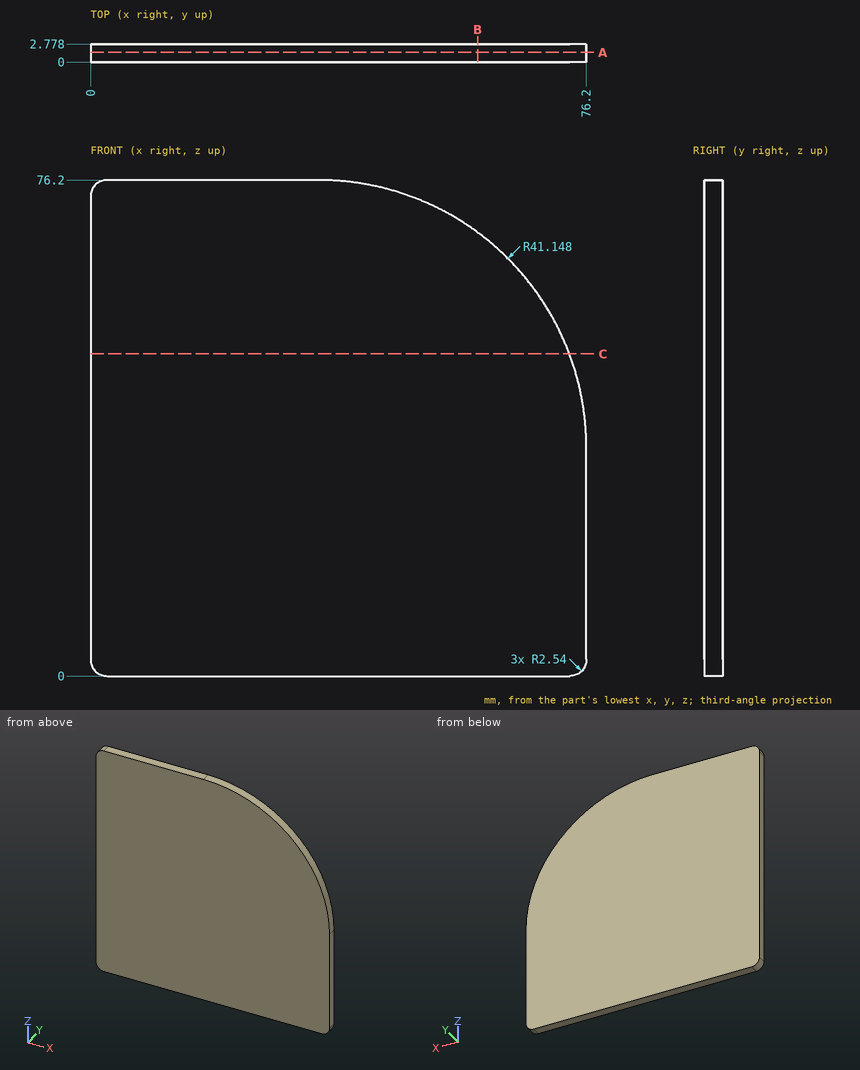
Answer from the drawing. Dimensions are ordinates in mm from the lowest x, y and z of the part. Coordinates: 2 decimals unless noted, no trailing zeros. Order: outer loops, then holes, each group sorted by start corner. A loop starts at its lowest first (then second) coordinate and runs counter-clockwise, first axis right, second up. Notation, with made-up numbers: M 24.25,-0.75 L 59.25,-0.75 A22 ccw 59.25,10.25 Z; hole C 86.25,0 d5. An arc over 180 degrees is marked long. Put each result on its own line as item: value. Start each with the question number.
Item 1: Section C-C, the plane z = 49.5 is taken. Determine the outline of the cut face in (x, y).
Item 2: Section B-B, the plane x = 59.5 is taken. Determine the outline of the cut face in (y, z).
Item 3: Section A-A, the plane y = 1.5 is taken. Determine the outline of the cut face in (x, z), plus the area to 3 significant figures.
Item 4: Consider probe 1 along X at (y, z) = (1.6, 35.5); probe 2 along Z at (x, y) = (58, 0.4); probe 3 along X at (y, z) = (1.4, 54). Determine where each line is inside the solid, lowest interval first. Write a range as [from, to].
Computed:
1. outline: M 0,0 L 73.58,0 L 73.58,2.78 L 0,2.78 Z
2. outline: M 0,0 L 2.78,0 L 2.78,68.15 L 0,68.15 Z
3. outline: M 0,2.54 A2.54 ccw 2.54,0 L 73.66,0 A2.54 ccw 76.2,2.54 L 76.2,35.05 A41.15 ccw 35.05,76.2 L 2.54,76.2 A2.54 ccw 0,73.66 Z
3. area: 5,440 mm2
4. probe 1: x = [0, 76.2]
4. probe 2: z = [0, 69.21]
4. probe 3: x = [0, 71.58]
